from build123d import *

# Parameters (mm, degrees)
BOSS_EXTRUDE1_START             = 199.569918
SKETCH6_R                       = 10.9982
BOSS_EXTRUDE1_DEPTH             = 6.35
F_5_0MM_DOWEL_HOLE2_D           = 5
F_5_0MM_DOWEL_HOLE2_DEPTH       = 25.4
F_5_0MM_DOWEL_HOLE2_CSINK_D     = 5.05
F_5_0MM_DOWEL_HOLE2_CSINK_ANGLE = 90
F_5_0MM_DOWEL_HOLE2_TIP         = 1.502151548
F_5_0MM_DOWEL_HOLE3_D           = 5
F_5_0MM_DOWEL_HOLE3_DEPTH       = 25.4
F_5_0MM_DOWEL_HOLE3_CSINK_D     = 5.05
F_5_0MM_DOWEL_HOLE3_CSINK_ANGLE = 90
F_5_0MM_DOWEL_HOLE3_TIP         = 1.502151548


with BuildPart() as part:
    # Sketch6 → Boss-Extrude1 (new body)
    with BuildSketch(Plane(origin=(0, 0, 0), x_dir=(0, 0, -1), z_dir=(1, 0, 0)).offset(BOSS_EXTRUDE1_START)):
        Polygon((74.6125, 36.5633), (128.5875, 36.5633), (128.5875, 96.52), (114.3, 96.52), (114.3, 76.2), (88.9, 76.2), (88.9, 96.52), (74.6125, 96.52), align=None)
        with Locations((101.6, 54.0258)):
            Circle(SKETCH6_R, mode=Mode.SUBTRACT)
    extrude(amount=-BOSS_EXTRUDE1_DEPTH)

    # Ø5.0mm Dowel Hole2
    with Locations(Plane.ZY.offset(-193.219917581)):
        with Locations((-101.6, 68.3133), (-87.3125, 54.0258), (-101.6, 39.7383), (-115.8875, 54.0258)):
            CounterSinkHole(F_5_0MM_DOWEL_HOLE2_D / 2, F_5_0MM_DOWEL_HOLE2_CSINK_D / 2, depth=F_5_0MM_DOWEL_HOLE2_DEPTH, counter_sink_angle=F_5_0MM_DOWEL_HOLE2_CSINK_ANGLE)
            with Locations((0, 0, -(F_5_0MM_DOWEL_HOLE2_DEPTH + F_5_0MM_DOWEL_HOLE2_TIP / 2))):  # 118° drill point
                Cone(0, F_5_0MM_DOWEL_HOLE2_D / 2, F_5_0MM_DOWEL_HOLE2_TIP, mode=Mode.SUBTRACT)

    # Ø5.0mm Dowel Hole3
    with Locations(Plane(origin=(0, 96.52, 0), x_dir=(1, 0, 0), z_dir=(0, 1, 0))):
        with Locations((196.394917581, 80.9625), (196.394917581, 122.2375)):
            CounterSinkHole(F_5_0MM_DOWEL_HOLE3_D / 2, F_5_0MM_DOWEL_HOLE3_CSINK_D / 2, depth=F_5_0MM_DOWEL_HOLE3_DEPTH, counter_sink_angle=F_5_0MM_DOWEL_HOLE3_CSINK_ANGLE)
            with Locations((0, 0, -(F_5_0MM_DOWEL_HOLE3_DEPTH + F_5_0MM_DOWEL_HOLE3_TIP / 2))):  # 118° drill point
                Cone(0, F_5_0MM_DOWEL_HOLE3_D / 2, F_5_0MM_DOWEL_HOLE3_TIP, mode=Mode.SUBTRACT)


solid = part.part
Can you work these out from the model? Positions are in its coordinate system, mm. A direction names the side the tool comes from. Give positions to 0.01 mm unless a question says otherwise; leave off trailing zeros. Loops run counter-clockwise (first coordinate to the right, second up) from the corner with the lowest first, then second, coordinate; pieces in that order, holes last. Notation, with made-up numbers: (89.5, 7) - (133.5, 7) arc R17 cw to (133.5, 15) - close; hole circle Ø10 at (33.5, -28). An arc over 180 degrees is marked (long way). Return JSON: item names as keys, results as strings.
1. I want a section at B-B on z = -101.6. Give the number of separate pieces and of enclosed holes in the cut face, and give its area (3 significant figures).
Output values:
{"separate pieces": "4", "enclosed holes": "0", "area": "48.5 mm²"}
2. I want a section at C-C on y = 46. Please give me the cut outline in (x, z), and give its area (3 significant figures).
Output values:
{"outline": "(193.22, -128.59) - (199.57, -128.59) - (199.57, -109.12) - (193.22, -109.12) - close; (193.22, -94.08) - (199.57, -94.08) - (199.57, -74.61) - (193.22, -74.61) - close", "area": "247 mm²"}
3. I'm going to push flat-ended pins straight in: pin 1 Ø1 at (x, z) = (195.5, -96.5) entering from +Y; pin 2 Ø4 at (y, z) = (54.03, -115.89) entering from -X. Where does each tip first touch, or does it pass through?
Output values:
{"pin 1": "stops at y = 76.2", "pin 2": "passes through"}
4. I want a section at A-A on y = 78. Please give me the cut outline in (x, z).
Output values:
{"outline": "(193.22, -128.59) - (199.57, -128.59) - (199.57, -114.3) - (193.22, -114.3) - close; (193.22, -88.9) - (199.57, -88.9) - (199.57, -74.61) - (193.22, -74.61) - close; hole circle Ø5 at (196.39, -122.24); hole circle Ø5 at (196.39, -80.96)"}
5. For faces 1 (the face through (196, 87, -114.3)), 2 (the face through (194.086, 83.63, -121.28)), 3 (the face through (197.9, 96.52, -83.4)), which set-ups out of +Z, -Z, +X, -X, +Y, -Y let a thin tool reach every point of the face, with its end or its side?
Output values:
{"face 1": "+X, -X, +Y", "face 2": "+Y", "face 3": "+Z, -Z, +X, -X, +Y"}
6. If I drill on line 1 (Y direction, x = 195.75, z = -101.6); line 2 (Z direction, x = 194.5, y = 82); line 3 (Y direction, x = 195.75, z = -102.5), over which ranges is the centre line in solid material (lowest first)?
Output values:
{"line 1": "y = 36.56 to 37.24, 42.24 to 43.03, 65.02 to 65.81, 70.81 to 76.2", "line 2": "z = -128.59 to -123.87, -120.61 to -114.3, -88.9 to -82.59, -79.33 to -74.61", "line 3": "y = 36.56 to 37.41, 42.07 to 43.06, 64.99 to 65.98, 70.65 to 76.2"}
7. We'd pull the mould along X, two halves only. Please class faces 4 (the face through (196, 36.563, -101)), 5 (the face through (194.086, 83.63, -80.005)): +X half, -X half, draft (parallel to the pull), parting line (faces both ways), or undercut.
Output values:
{"face 4": "draft", "face 5": "undercut"}
8. I want a section at D-D on z = -110. Please give me the cut outline in (x, y).
Output values:
{"outline": "(193.22, 36.56) - (199.57, 36.56) - (199.57, 46.93) - (193.22, 46.93) - close; (193.22, 61.13) - (199.57, 61.13) - (199.57, 76.2) - (193.22, 76.2) - close"}
